from build123d import *

# Parameters (mm, degrees)
F1_DEPTH = 25
F2_W     = 75
F2_H     = 15
F2_W_2   = 25
F3_DEPTH = 7
F4_R     = 5
F6_W     = 50
F6_H     = 20
F6_W_2   = 25
F7_DEPTH = 7
F8_R     = 10


with BuildPart() as f1:
    # F0 (on Right) → F1 (new body)
    with BuildSketch(Plane.YZ):
        with BuildLine():
            ThreePointArc((-25.1164593902, -17.3035680626), (0, 30.5), (25.1164593902, -17.3035680626))
            Line((25.1164593902, -17.3035680626), (28.0068792885, -23.275158049))
            ThreePointArc((28.0068792885, -23.275158049), (34.7936009681, 10.7481906084), (10, 35.015971637))
            Line((10, 35.015971637), (-10, 35.015971637))
            ThreePointArc((-10, 35.015971637), (-34.7936009681, 10.7481906084), (-28.0068792885, -23.275158049))
            Line((-28.0068792885, -23.275158049), (-25.1164593902, -17.3035680626))
        make_face()
    extrude(amount=F1_DEPTH)

    # F4
    f4_edges = [f1.edges().sort_by_distance(p)[0] for p in [
        (0, -26.561669, -20.289363),
        (12.5, 25.116459, -17.303568),
        (12.5, -25.116459, -17.303568),
        (0, 26.561669, -20.289363),
    ]]
    fillet(f4_edges, radius=F4_R)

    # F6 (on face) → F7 (join)
    with BuildSketch(Plane.XY.offset(35.015971637)):
        with Locations((-25, 0)):
            Rectangle(F6_W, F6_H)
        with Locations((12.5, 0)):
            Rectangle(F6_W_2, F6_H)
    extrude(amount=F7_DEPTH)

    # F8
    f8_edges = [f1.edges().sort_by_distance(p)[0] for p in [
        (12.5, -10, 35.015972),
        (12.5, 10, 35.015972),
    ]]
    fillet(f8_edges, radius=F8_R)


with BuildPart() as f3:
    # F2 (on face) → F3 (new body)
    with BuildSketch(Plane.XY.offset(35.015971637)):
        with Locations((-37.5, 0)):
            Rectangle(F2_W, F2_H)
        with Locations((12.5, 0)):
            Rectangle(F2_W_2, F2_H)
    extrude(amount=F3_DEPTH)


solid = f1.part
Check sheet for the modelled part. Datum: model origin and axes. Units: mm. A direction names the side the tool comes from. Give positions to 0.01 mm unless a question says otherwise; leave off trailing zeros. Write each loop counter-clockwise with the first axis right and the second up, starting at its lowest first coordinate (ties: lowest second). Pieces come first, ordered by that corner, then holes. Notation, with made-up numbers: (57, 2) -> (70, 2) arc R10 cw to (70, 11) -> close; hole circle Ø11 at (-24.5, -15). An arc over 180 degrees is marked (long way). One line per item, written item: value. Start each with the question number.
Item 1: Section check A-A on z = 0. Record the cut outline in (x, y), then the cut area to 3 significant figures.
Item 2: Section check C-C on z = 16. Record the cut outline in (x, y), then the cut area to 3 significant figures.
Item 3: Draft check along Z on faces 5 (the cylindrical face through (13.107, -25.826, -17.409)), 6 (the cylindrical face through (12.68, -11.5, 36.62)), 7 (the cylindrical face through (12.325, -35.468, 8.256)). Enter one of: +Z half, -Z half, draft (parallel to the pull), parting line (faces both ways), or undercut.
Item 4: Gauge pin test, flat ends, axial feed: pin 1 (5 mm diameter, centred on y = -15, z = 31, fed in from -X); pin 2 (3 mm diameter, centred on x = -34, y = 12.5, fed in from +Z); pin 3 (3.5 mm diameter, centred on x = -31, z = 39.5, fed in from +Y); pin 4 (16 mm diameter, centred on x = -19, y = 1.5, fed in from -Z). Record the tip position at first contact, or that the pin passes through.
Item 5: Material ranges on probe 1 along Y at (x, z) = (10.25, 0); probe 2 along Z at (x, y) = (9.5, 0); probe 3 along X at (y, z) = (16.5, 28.5), recorded low to high. Write a range as from..to.
Item 6: Section check D-D on x = -19.5. Record the cut outline in (y, z).
Item 7: Section check B-B on y = 0. Record the cut outline in (x, z).
Item 8: Tool access check on faces 1 (the cylindrical face through (1.5, 27.6, -19.15)), 2 (the flat face through (14.86, 27.152, -21.51)), 3 (the cylindrical face through (13.107, 25.826, -17.409)), 4 (the flat face through (-25, 0, 35.016)). Record the directions out of +Z, -Z, +X, -X, +Y, -Y that give a thin tool (end or side, any length) a straight path to the whole face; none if there is none.
Results list:
1. outline: (0, -36.42) -> (25, -36.42) -> (25, -30.5) -> (0, -30.5) -> close; (0, 30.5) -> (25, 30.5) -> (25, 36.42) -> (0, 36.42) -> close
1. area: 296 mm²
2. outline: (0, -32.71) -> (25, -32.71) -> (25, -25.97) -> (0, -25.97) -> close; (0, 25.97) -> (25, 25.97) -> (25, 32.71) -> (0, 32.71) -> close
2. area: 337 mm²
3. face 5: undercut
3. face 6: +Z half
3. face 7: parting line
4. pin 1: x = 0
4. pin 2: through
4. pin 3: y = 10
4. pin 4: z = 35.02
5. probe 1: -36.42..-30.5, 30.5..36.42
5. probe 2: 30.5..42.02
5. probe 3: 0..25
6. outline: (-10, 35.02) -> (10, 35.02) -> (10, 42.02) -> (-10, 42.02) -> close
7. outline: (-50, 35.02) -> (0, 35.02) -> (0, 30.5) -> (25, 30.5) -> (25, 42.02) -> (-50, 42.02) -> close
8. face 1: -Z, -X
8. face 2: -Z, +X, -X
8. face 3: +X, -X
8. face 4: -Z, -X, +Y, -Y
